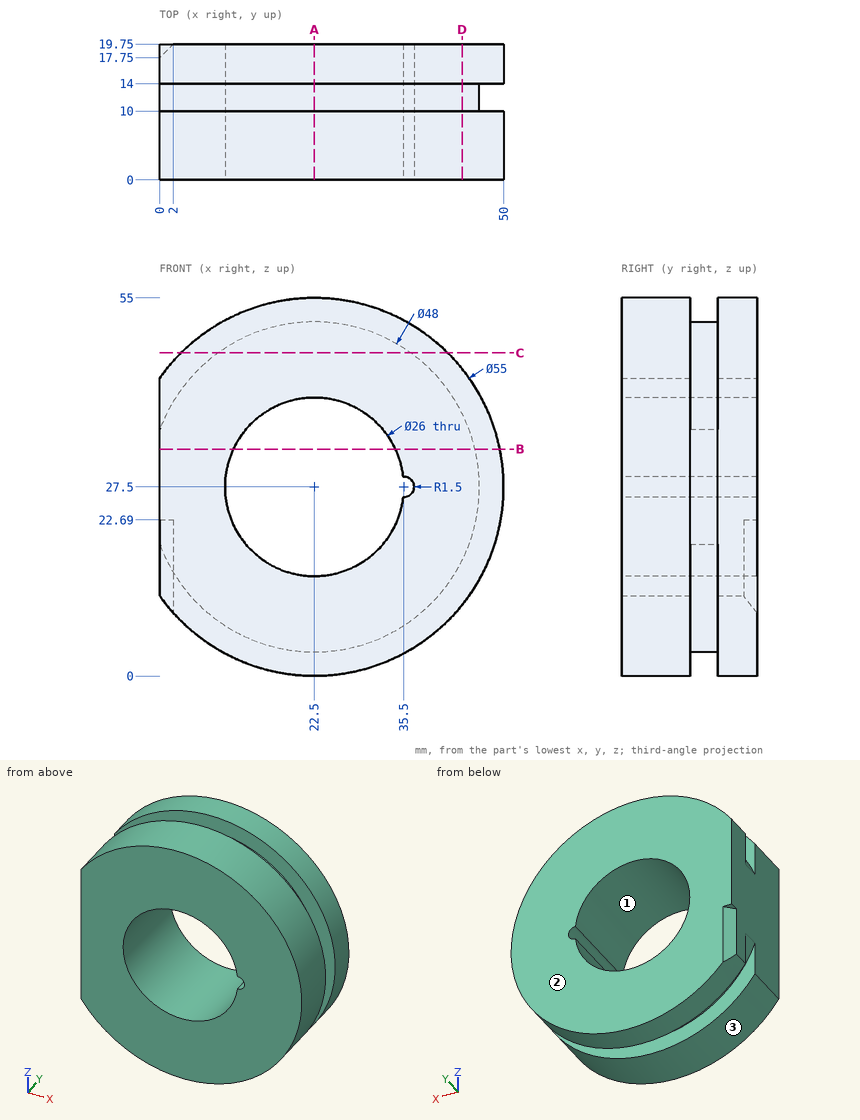
Drawing for the job (mm, zero at the part's lowest x, y, z). Give positions to 0.01 mm unless a question says otherwise; leave off trailing zeros. Write each loop counter-clockwise with the first axis right and the second up, starting at its lowest first coordinate (ties: lowest second). Pieces come first, ordered by that corner, then holes. Notation, with made-up numbers: (51, 73) -> (110, 73) arc R21 ccw to (110, 82) -> close; hole circle Ø5 at (67, 75.5). An arc over 180 degrees is marked (long way). Put each result on its own line as item: value. Start each with the question number.
Item 1: Cut at C-C (z = 47). List the corners of the cut face in (x, y).
Item 2: Wall check: L1, parallel to Y at x = 31, z = 52.5; L2, parallel to Z at x = 22.5, y = 5.25; L3, parallel to Z at x = 22.5, y = 10.25. Give the ranges that are in metal, low to high. Write a range as [from, to].
Item 3: Cut at B-B (z = 33). List the corners of the cut face in (x, y).
Item 4: Pull direction Z, two halves, no side cores. Call the marked faces 1, 2 and 3: pulls with the +Z half, pulls with the -Z half, needs draft (parallel to the pull), parting line crosses it, or undercut.
Item 5: Cut at D-D (x = 44). List the corners of the cut face in (y, z), then the cut area to 3 significant figures.
Item 6: Pin check, flat tips, straight feed: pin 1 Ø6 at (x, y) = (41.5, 5.5) entering from +Z; pin 2 Ø1 at (x, y) = (25, 4) entering from +Z; pin 3 Ø1.6 at (x, y) = (1, 19) entering from -Z. Stop position of each tip, or through.
Item 7: Cut at A-A (x = 22.5). List the corners of the cut face in (y, z).
Answer list:
1. outline: (3.11, 0) -> (41.89, 0) -> (41.89, 10) -> (36.49, 10) -> (36.49, 14) -> (41.89, 14) -> (41.89, 19.75) -> (3.11, 19.75) -> (3.11, 14) -> (8.51, 14) -> (8.51, 10) -> (3.11, 10) -> close
2. L1: y = [0, 10], [14, 19.75]
2. L2: z = [0, 14.5], [40.5, 55]
2. L3: z = [3.5, 14.5], [40.5, 51.5]
3. outline: (0, 0) -> (10.72, 0) -> (10.72, 19.75) -> (0, 19.75) -> close; (34.28, 0) -> (49.44, 0) -> (49.44, 10) -> (45.86, 10) -> (45.86, 14) -> (49.44, 14) -> (49.44, 19.75) -> (34.28, 19.75) -> close
4. face 1: undercut
4. face 2: needs draft
4. face 3: parting line crosses it
5. outline: (0, 10.35) -> (10, 10.35) -> (10, 16.83) -> (14, 16.83) -> (14, 10.35) -> (19.75, 10.35) -> (19.75, 44.65) -> (14, 44.65) -> (14, 38.17) -> (10, 38.17) -> (10, 44.65) -> (0, 44.65) -> close
5. area: 625 mm2
6. pin 1: stops at z = 49.87
6. pin 2: stops at z = 54.93
6. pin 3: stops at z = 9.4
7. outline: (0, 0) -> (10, 0) -> (10, 3.5) -> (14, 3.5) -> (14, 0) -> (19.75, 0) -> (19.75, 14.5) -> (0, 14.5) -> close; (0, 40.5) -> (19.75, 40.5) -> (19.75, 55) -> (14, 55) -> (14, 51.5) -> (10, 51.5) -> (10, 55) -> (0, 55) -> close
